Design review of the part built by this model. Coordinates are the model's own, in mm. Round coordinates to 2 decimals unless told otherwise and drop trailing zeros. Loops run counter-clockwise (first coordinate to the right, second up) from the corner with the lowest first, then second, coordinate; pieces in that order, holes last. Notation, with made-up numbers: (27, 85.25) -> (37, 85.25) arc R16 ccw to (37, 102.25) -> close; hole circle Ø7 at (86.5, -4). An arc over 180 degrees is marked (long way). Answer as CSV lines item,"result". Start each with the question number.
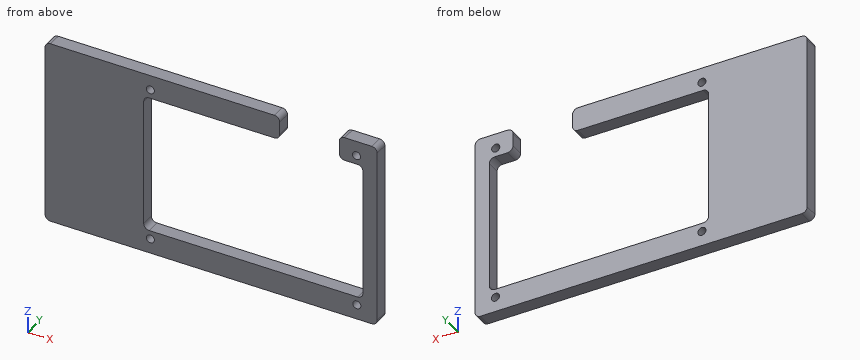
Autodesk Inventor part; units mm, degrees
ref_plane "YZ Plane" through (0, 0, 0) normal (1, 0, 0) x (0, 1, 0)
ref_plane "XZ Plane" through (0, 0, 0) normal (0, 1, 0) x (-1, 0, 0)
ref_plane "XY Plane" through (0, 0, 0) normal (0, 0, 1) x (1, 0, 0)
sketch "Sketch1" plane through (0, 0, 0) normal (0, 1, 0) x (-1, 0, 0)
  line L0 (-2.27, 0) -> (120.44, 0)
  line L1 (120.44, 0) -> (120.44, -68.57)
  line L2 (120.44, -68.57) -> (-2.27, -68.57)
  line L3 (-2.27, -68.57) -> (-2.27, 0)
  line L4 (120.44, -66.57) -> (120.44, -2)
  line L5 (0, -68.57) -> (118.44, -68.57)
  line L6 (-2.27, -2.27) -> (-2.27, -66.3)
  circle A0 centre (81.55, -63.09) radius 1.5
  circle A1 centre (81.55, -63.09) radius 1.5
  line L7 (70.44, -68.57) -> (15.73, -68.57)
  line L8 (51, 0) -> (75, 0)
  line L9 (26, 0) -> (51, 0)
  line L10 (84, -60) -> (79, -60)
  line L11 (79, -60) -> (79, -8.7337)
  line L12 (79, -8.7337) -> (84, -8.7337)
  line L13 (84, -8.7337) -> (84, -60)
  line L14 (8, -60) -> (3, -60)
  line L15 (3, -60) -> (3, -8.7337)
  line L16 (3, -8.7337) -> (8, -8.7337)
  line L17 (8, -8.7337) -> (8, -60)
  circle A2 centre (5.25, -63.09) radius 1.5
  circle A3 centre (5.35, -5.47) radius 1.5
  circle A4 centre (81.55, -5.47) radius 1.5
  circle A5 centre (81.55, -5.47) radius 1.5
  circle A6 centre (5.35, -5.47) radius 1.5
  circle A7 centre (5.25, -63.09) radius 1.5
  dimension "d20" = 3
  dimension "d27" = 3
  dimension "d28" = 3
  dimension "d29" = 3
  dimension "d30" = 68.57
extrude "Extrusion1" add sketch "Sketch1" along normal blind 5
fillet "Fillet4" radius 2 4 edges at (-120.44, 2.5, -68.57) (-120.44, 2.5, 0) (2.27, 2.5, -68.57) (2.27, 2.5, 0)
sketch "Sketch7" plane through (0, 5, 0) normal (0, 1, 0) x (1, 0, 0)
  line L0 (-117.44, 63.57) -> (-87.44, 63.57)
  line L1 (-87.44, 63.57) -> (-87.44, 5)
  line L2 (-87.44, 5) -> (-117.44, 5)
  line L3 (-117.44, 5) -> (-117.44, 63.57)
  line L4 (-120.44, 66.57) -> (-120.44, 2)
  line L5 (0.27, 68.57) -> (-118.44, 68.57)
  line L6 (-118.44, 0) -> (0.27, 0)
  point P0 (0, 0)
  dimension "d67" = 30
  dimension "d68" = 3
  dimension "d69" = 5
  dimension "d70" = 5
extrude "Extrusion6" [suppressed]
fillet "Fillet8" [suppressed]
sketch "Sketch8" plane through (0, 5, 0) normal (0, 1, 0) x (1, 0, 0)
  line L0 (-79, 60) -> (-8, 60)
  line L1 (-8, 60) -> (-8, 8.7337)
  line L2 (-8, 8.7337) -> (-79, 8.7337)
  line L3 (-79, 8.7337) -> (-79, 60)
  line L4 (-8, 8.7337) -> (-8, 60)
  line L5 (0.27, 68.57) -> (-118.44, 68.57)
  line L6 (-79, 60) -> (-79, 8.7337)
  line L7 (-3, 8.7337) -> (-8, 8.7337)
  line L8 (-8, 60) -> (-3, 60)
  point P0 (0, 0)
extrude "Extrusion7" cut sketch "Sketch8" against normal blind 10
sketch "Sketch9" plane through (0, 5, 0) normal (0, 1, 0) x (1, 0, 0)
  line L0 (-3, 8.7337) -> (-84, 8.7337)
  line L1 (-118.44, 0) -> (0.27, 0)
  line L2 (-33.73, 8.7337) -> (-11.73, 8.7337)
  line L3 (-11.73, 8.7337) -> (-11.73, 0)
  line L4 (-11.73, 0) -> (-33.73, 0)
  line L5 (-33.73, 0) -> (-33.73, 8.7337)
  line L6 (2.27, 2) -> (2.27, 66.57)
  point P0 (0, 0)
  point P1 (-79, 8.57)
  point P2 (-8, 8.57)
  point P3 (-33.73, 0)
  point P4 (-11.73, 8.57)
  point P5 (-11.73, 8.7337)
  point P6 (-79, 8.871)
  point P7 (-8, 8.871)
  point P8 (-11.73, 8.871)
  point P9 (-11.73, 8.7337)
  dimension "d78" = 22
  dimension "d81" = 14
  dimension "d82" = 8.7338
extrude "Extrusion8" cut sketch "Sketch9" against normal blind 5
fillet "Fillet9" radius 2 8 edges at (-84, 2.5, -60) (-3, 2.5, -60) (-3, 2.5, -8.7337) (-11.73, 2.5, -8.7337) (-11.73, 2.5, 0) (-33.73, 2.5, -8.7337) (-33.73, 2.5, 0) (-84, 2.5, -8.7337)
properties part number "Top PMMA"
Q1. For pin 1 Ø2.5 at (x, z) = (-81.55, -5.47) entering from +Y, flat-tipped, find the tip position at first contact; note if it passes through.
Q2. Add section A-A, the plane z = -49.5. Give the boundary of the cut face in (x, y), and give its area (3 significant figures).
Q3. Add section B-B, the plane z = -5.47. Give the boundary of the cut face in (x, y).
Q4. To check wall thickness, follow probe 1 along Z at (x, y) = (-81.55, 3.9); probe 2 along X at (y, z) = (0.75, -24); probe 3 along X at (y, z) = (1.45, -6.5). State the ranges of each line that lie inside material, in increasing order. Write a range as from..to.
Q5. Add section D-D, the plane x = -52.5. Give the boundary of the cut face in (y, z).
Q6. Add section C-C, the plane y = 3.9. Give the boundary of the cut face in (x, z), and give its area (3 significant figures).
Worked answers:
1,pin 1,"passes through"
2,outline,"(-120.44, 0) -> (-84, 0) -> (-84, 5) -> (-120.44, 5) -> close; (-3, 0) -> (2.27, 0) -> (2.27, 5) -> (-3, 5) -> close"
2,area,"209 mm^2"
3,outline,"(-120.44, 0) -> (-83.05, 0) -> (-83.05, 5) -> (-120.44, 5) -> close; (-80.05, 0) -> (-33.73, 0) -> (-33.73, 5) -> (-80.05, 5) -> close; (-11.73, 0) -> (-6.85, 0) -> (-6.85, 5) -> (-11.73, 5) -> close; (-3.85, 0) -> (2.27, 0) -> (2.27, 5) -> (-3.85, 5) -> close"
4,probe 1,"z = -68.57..-64.59, -61.59..-60, -8.73..-6.97, -3.97..0"
4,probe 2,"x = -120.44..-84, -3..2.27"
4,probe 3,"x = -120.44..-82.64, -80.46..-33.73, -11.73..-6.44, -4.26..2.27"
5,outline,"(0, -68.57) -> (5, -68.57) -> (5, -60) -> (0, -60) -> close; (0, -8.73) -> (5, -8.73) -> (5, 0) -> (0, 0) -> close"
6,outline,"(-120.44, -66.57) arc R2 ccw to (-118.44, -68.57) -> (0.27, -68.57) arc R2 ccw to (2.27, -66.57) -> (2.27, -2) arc R2 ccw to (0.27, 0) -> (-9.73, 0) arc R2 ccw to (-11.73, -2) -> (-11.73, -6.73) arc R2 ccw to (-9.73, -8.73) -> (-5, -8.73) arc R2 cw to (-3, -10.73) -> (-3, -58) arc R2 cw to (-5, -60) -> (-82, -60) arc R2 cw to (-84, -58) -> (-84, -10.73) arc R2 cw to (-82, -8.73) -> (-35.73, -8.73) arc R2 ccw to (-33.73, -6.73) -> (-33.73, -2) arc R2 ccw to (-35.73, 0) -> (-118.44, 0) arc R2 ccw to (-120.44, -2) -> close; hole circle Ø3 at (-81.55, -63.09); hole circle Ø3 at (-81.55, -5.47); hole circle Ø3 at (-5.35, -5.47); hole circle Ø3 at (-5.25, -63.09)"
6,area,"4,040 mm^2"
